Can you work these out from the model? Positions are in its coordinate system, mm. A direction names the side the tool comes from. Round coordinates to 2 decimals unless told otherwise and drop trailing zeros. Write each loop counter-clockwise with the first axis right and the second up, starting at its lowest first coordinate (ties: lowest second). Pieces come first, ordered by that corner, then holes. Notation, with made-up numbers: (61.5, 36) - (114.5, 36) arc R19 ccw to (114.5, 54) - close; hole circle Ø5 at (77, 54). An arc over 180 degrees is marked (long way). One line per item, written item: value. Start each with the question number.
(1) If I drill on L1, parallel to Y at x = 0.1, z = 0; L2, parallel to Z at x = 0.05, y = 8.25, over which ranges is the centre line in solid material (lowest first)? Write a range as from..to.
(2) I want a section at C-C on y = 9. List the corners of the cut face in (x, z) for me.
(3) On a 3-axis mill with a long thin cutter (end or side, diameter ignored), from which of +Z, -Z, +X, -X, +Y, -Y can I reach the whole of each face in a straight line? I mean faces 1 (the face through (-0.581, 12.796, 0.302)), 2 (the face through (0.506, 5.701, 0.323)), 3 (the face through (0, 14, 0)). Say none if no direction works.
(4) I want a section at B-B on y = 13. List the corners of the cut face in (x, z) for me (3 decimals), plus the area to 3 significant figures.
from build123d import *

# Parameters (mm, degrees)
SKETCH1_R           = 0.6
BOSS_EXTRUDE1_DEPTH = 11.45
CHAMFER1_SIZE       = 0.25
SKETCH3_R           = 0.85
BOSS_EXTRUDE2_DEPTH = 0.15
SKETCH4_R           = 0.655
BOSS_EXTRUDE3_DEPTH = 2.95
SKETCH5_W           = 0.965055555
SKETCH5_H           = 1.860066756
CUT_EXTRUDE1_DEPTH  = 1.25
CHAMFER2_SIZE       = 0.195
CHAMFER2_SIZE_2     = 0.112583302
CHAMFER3_SIZE       = 0.144
CHAMFER3_SIZE2      = 0.249415316


with BuildPart() as part:
    # Sketch1 → Boss-Extrude1 (new body)
    with BuildSketch(Plane(origin=(0, 0, 0), x_dir=(1, 0, 0), z_dir=(0, 1, 0))):
        with Locations(Location((0, 0, 0), (0, 0, 270))):
            Circle(SKETCH1_R)
    extrude(amount=BOSS_EXTRUDE1_DEPTH)

    # Chamfer1
    chamfer1_edges = [part.edges().sort_by_distance(p)[0] for p in [
        (0, 0, -0.6),
    ]]
    chamfer(chamfer1_edges, length=CHAMFER1_SIZE)

    # Sketch3 → Boss-Extrude2 (add)
    with BuildSketch(Plane(origin=(0, 11.45, 0), x_dir=(1, 0, 0), z_dir=(0, 1, 0))):
        with Locations(Location((0, 0, 0), (0, 0, 270))):
            Circle(SKETCH3_R)
    extrude(amount=BOSS_EXTRUDE2_DEPTH)

    # Sketch4 → Boss-Extrude3 (add)
    with BuildSketch(Plane(origin=(0, 11.6, 0), x_dir=(1, 0, 0), z_dir=(0, 1, 0))):
        with Locations(Location((0, 0, 0), (0, 0, 270))):
            Circle(SKETCH4_R)
    extrude(amount=BOSS_EXTRUDE3_DEPTH)

    # Sketch5 → Cut-Extrude1 (cut)
    with BuildSketch(Plane(origin=(0, 14.55, 0), x_dir=(1, 0, 0), z_dir=(0, 1, 0))):
        with Locations((0.482527778, -0.010701221)):
            Rectangle(SKETCH5_W, SKETCH5_H)
    extrude(amount=-CUT_EXTRUDE1_DEPTH, mode=Mode.SUBTRACT)

    # Chamfer2
    # the kernel refuses this chamfer: 0.195, 0.112583302 mm, written as the material it adds along each edge
    with BuildSketch(Plane(origin=(0, 11.6, 0), x_dir=(0, 0, 1), z_dir=(-1, 0, 0))) as chamfer2_piece_1_section:
        Polygon((0.655 + CHAMFER2_SIZE, 0), (0.655, CHAMFER2_SIZE_2 * 1.00000000437), (0.655, 0), align=None)
    chamfer2_piece_1 = revolve(axis=Axis((0, 11.6, 0), (0, 1, 0)), mode=Mode.PRIVATE)
    chamfer2_piece_1 = chamfer2_piece_1 & Plane(origin=(0, 11.654924412, 0), x_dir=(0, 0, 1), z_dir=(0, -1, 0)) * Cylinder(0.85, 4, mode=Mode.PRIVATE)
    add(chamfer2_piece_1)

    # Chamfer3
    chamfer3_edges = [part.edges().sort_by_distance(p)[0] for p in [
        (0, 11.45, -0.6),
    ]]
    chamfer3_side = [part.faces().sort_by_distance(p)[0] for p in [
        (0, 5.85, -0.6),
    ]]
    chamfer(chamfer3_edges, length=CHAMFER3_SIZE, length2=CHAMFER3_SIZE2, reference=chamfer3_side[0])


solid = part.part
Established:
1. L1: 0..13.3
1. L2: -0.6..0.6
2. outline: circle Ø1.2 at (0, 0)
3. face 1: +Y
3. face 2: -Y
3. face 3: +Z, -Z, +X, +Y
4. outline: circle Ø1.31 at (0, 0)
4. area: 1.35 mm2
